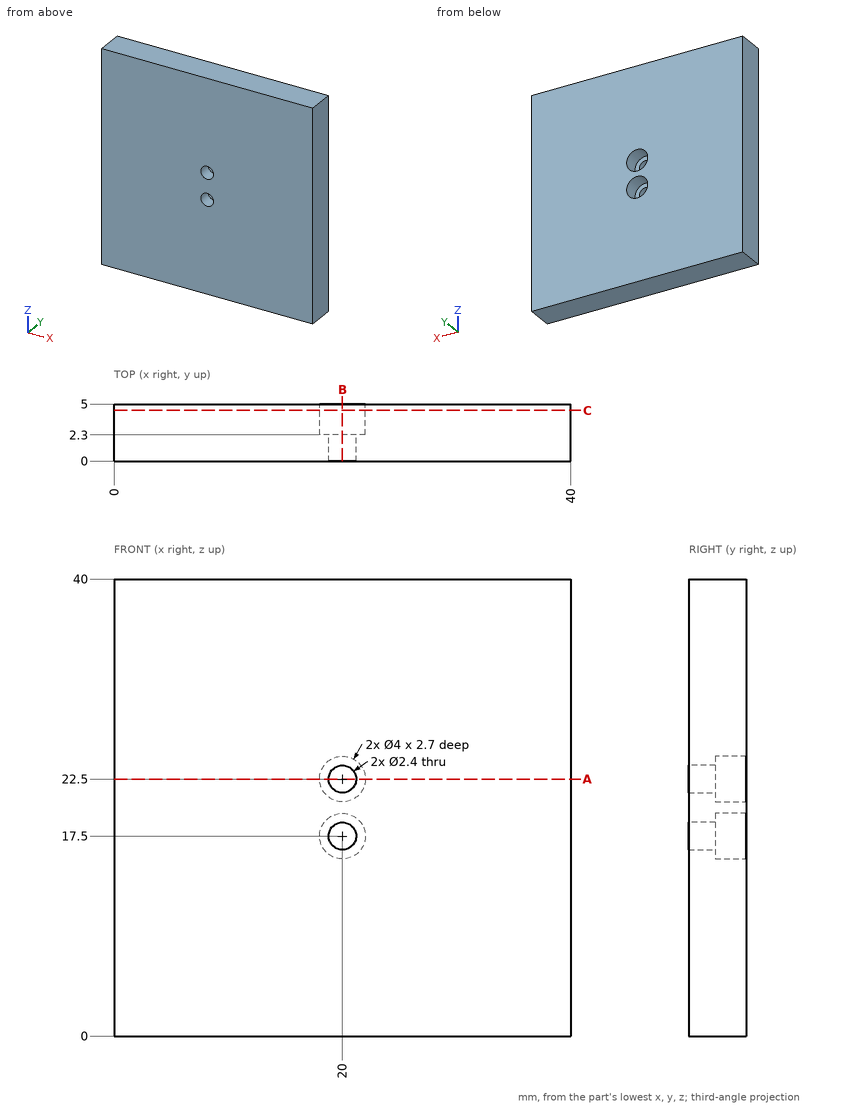
Job drawing, mm, ordinate dimensions from the low corner. One solid piece. Coordinates: 2 decimals unless noted, no trailing zeros. Loops run counter-clockwise (first coordinate to the right, second up) from the corner with the lowest first, then second, coordinate; pieces in that order, holes last. Notation, with made-up numbers: (68.5, 29) - (108.5, 29) arc R11 cw to (108.5, 40) - close; hole circle Ø5 at (18.5, 1.5). An arc over 180 degrees is marked (long way). Answer as a JSON object with one key per item and string values. Group by question number.
(1) Cut at A-A (z = 22.5). Give the cut face in (x, y), then the cut area to 3 significant figures.
(2) Probe line 1 along X through (y, z) = (3.1, 22.5); line 2 along X through (y, z) = (1.65, 17.5). List the from-to ranges inside material, lowest first.
(3) Cut at C-C (y = 4.45). Give the cut face in (x, z).
(4) Cut at B-B (x = 20). Give the cut face in (y, z), then the cut area to 3 significant figures.
(5) Flat gauge pins, fed straight in: pin 1 (1.4 mm diameter, centred on x = 20, z = 17.5, fed in from -Y); pin 2 (3.5 mm diameter, centred on x = 20, z = 17.5, fed in from +Y). Where does each tip first touch, or does it go through?
Geometry says:
{
 "1": {"outline": "(0, 0) - (18.8, 0) - (18.8, 2.3) - (18, 2.3) - (18, 5) - (0, 5) - close; (21.2, 0) - (40, 0) - (40, 5) - (22, 5) - (22, 2.3) - (21.2, 2.3) - close", "area": "184 mm^2"},
 "2": {"line 1": "x = 0 to 18, 22 to 40", "line 2": "x = 0 to 18.8, 21.2 to 40"},
 "3": {"outline": "(0, 0) - (40, 0) - (40, 40) - (0, 40) - close; hole circle Ø4 at (20, 17.5); hole circle Ø4 at (20, 22.5)"},
 "4": {"outline": "(0, 0) - (5, 0) - (5, 15.5) - (2.3, 15.5) - (2.3, 16.3) - (0, 16.3) - close; (0, 18.7) - (2.3, 18.7) - (2.3, 19.5) - (5, 19.5) - (5, 20.5) - (2.3, 20.5) - (2.3, 21.3) - (0, 21.3) - close; (0, 23.7) - (2.3, 23.7) - (2.3, 24.5) - (5, 24.5) - (5, 40) - (0, 40) - close", "area": "167 mm^2"},
 "5": {"pin 1": "passes through", "pin 2": "stops at y = 2.3"}
}
